from build123d import *

# Parameters (mm, degrees)
BOSS_EXTRUDE1_DEPTH = 15
BOSS_EXTRUDE2_DEPTH = 15
CUT_EXTRUDE1_DEPTH  = 14
SKETCH8_W           = 6.699223296
SKETCH8_H           = 4.721357371
SKETCH8_W_2         = 8.228893272
CUT_EXTRUDE7_DEPTH  = 3
SKETCH10_R          = 1.1
CUT_EXTRUDE9_DEPTH  = 15


with BuildPart() as part:
    # Sketch3 → Boss-Extrude1 (new body)
    with BuildSketch(Plane.XY.offset(1303.472903018)):
        with BuildLine():
            Line((787.650097371, 1035.49652121), (787.650097371, 1120.589424436))
            ThreePointArc((787.650097371, 1120.589424436), (788.529097371, 1122.710424436), (790.650097371, 1123.589424436))
            Line((790.650097371, 1123.589424436), (812.066097371, 1123.589424436))
            ThreePointArc((812.066097371, 1123.589424436), (814.187097371, 1122.710424436), (815.066097371, 1120.589424436))
            Line((815.066097371, 1120.589424436), (815.066097371, 1103.589424436))
            ThreePointArc((815.066097371, 1103.589424436), (815.945097371, 1101.468424436), (818.066097371, 1100.589424436))
            Line((818.066097371, 1100.589424436), (834.650097371, 1100.589424436))
            Line((834.650097371, 1100.589424436), (834.650461973, 1102.58942437))
            Line((834.650461973, 1102.58942437), (818.066461973, 1102.58942437))
            ThreePointArc((818.066461973, 1102.58942437), (817.35931084, 1102.882637905), (817.066097305, 1103.589789038))
            Line((817.066097305, 1103.589789038), (817.066097305, 1120.589789038))
            ThreePointArc((817.066097305, 1120.589789038), (815.601310896, 1124.124637961), (812.066461973, 1125.58942437))
            Line((812.066461973, 1125.58942437), (790.64973277, 1125.58942437))
            ThreePointArc((790.64973277, 1125.58942437), (787.114883847, 1124.124637961), (785.650097438, 1120.589789038))
            Line((785.650097438, 1120.589789038), (785.650097371, 1033.49652121))
            Line((785.650097371, 1033.49652121), (834.649003168, 1033.49652121))
            Line((834.649003168, 1033.49652121), (834.649003168, 1035.49652121))
            Line((834.649003168, 1035.49652121), (787.650097371, 1035.49652121))
        make_face()
    extrude(amount=BOSS_EXTRUDE1_DEPTH)

    # Sketch6 → Boss-Extrude2 (add)
    with BuildSketch(Plane.XY.offset(1303.472903018)):
        with BuildLine():
            Line((787.650097371, 1035.49652121), (834.649003168, 1035.49652121))
            Line((834.649003168, 1035.49652121), (844.649003168, 1035.49652121))
            Line((844.649003168, 1035.49652121), (844.650097371, 1100.589424436))
            Line((844.650097371, 1100.589424436), (834.650097371, 1100.589424436))
            Line((834.650097371, 1100.589424436), (818.066097371, 1100.589424436))
            ThreePointArc((818.066097371, 1100.589424436), (815.945097371, 1101.468424436), (815.066097371, 1103.589424436))
            Line((815.066097371, 1103.589424436), (815.066097371, 1120.589424436))
            ThreePointArc((815.066097371, 1120.589424436), (814.187097371, 1122.710424436), (812.066097371, 1123.589424436))
            Line((812.066097371, 1123.589424436), (790.650097371, 1123.589424436))
            ThreePointArc((790.650097371, 1123.589424436), (788.529097371, 1122.710424436), (787.650097371, 1120.589424436))
            Line((787.650097371, 1120.589424436), (787.650097371, 1035.49652121))
        make_face()
    extrude(amount=BOSS_EXTRUDE2_DEPTH)

    # Sketch6<2> → Cut-Extrude1 (cut)
    with BuildSketch(Plane.XY.offset(1303.472903018)):
        with BuildLine():
            Line((787.650097371, 1035.49652121), (834.649003168, 1035.49652121))
            Line((834.649003168, 1035.49652121), (844.649003168, 1035.49652121))
            Line((844.649003168, 1035.49652121), (844.650097371, 1100.589424436))
            Line((844.650097371, 1100.589424436), (834.650097371, 1100.589424436))
            Line((834.650097371, 1100.589424436), (818.066097371, 1100.589424436))
            ThreePointArc((818.066097371, 1100.589424436), (815.945097371, 1101.468424436), (815.066097371, 1103.589424436))
            Line((815.066097371, 1103.589424436), (815.066097371, 1120.589424436))
            ThreePointArc((815.066097371, 1120.589424436), (814.187097371, 1122.710424436), (812.066097371, 1123.589424436))
            Line((812.066097371, 1123.589424436), (790.650097371, 1123.589424436))
            ThreePointArc((790.650097371, 1123.589424436), (788.529097371, 1122.710424436), (787.650097371, 1120.589424436))
            Line((787.650097371, 1120.589424436), (787.650097371, 1035.49652121))
        make_face()
    extrude(amount=CUT_EXTRUDE1_DEPTH, mode=Mode.SUBTRACT)

    # Sketch8 → Cut-Extrude7 (cut)
    with BuildSketch(Plane.XY.offset(1303.472903018)):
        with Locations((788.177093813, 1120.255926572)):
            Rectangle(SKETCH8_W, SKETCH8_H)
        with Locations((813.958809837, 1120.255926572)):
            Rectangle(SKETCH8_W_2, SKETCH8_H)
    extrude(amount=CUT_EXTRUDE7_DEPTH, mode=Mode.SUBTRACT)

    # Sketch10 → Cut-Extrude9 (cut)
    with BuildSketch(Plane.XY.offset(1303.472903018)):
        with Locations((832.650097371, 1039.589424436)):
            Circle(SKETCH10_R)
        with Locations((792.650097371, 1039.589424436)):
            Circle(SKETCH10_R)
        with Locations((792.650097371, 1097.589424436)):
            Circle(SKETCH10_R)
        with Locations((812.650097371, 1097.589424436)):
            Circle(SKETCH10_R)
    extrude(amount=CUT_EXTRUDE9_DEPTH, mode=Mode.SUBTRACT)


solid = part.part
Could you check a few things on this model? Use its own coordinates, in mm. A direction names the side the tool comes from. Give positions to 0.01 mm unless a question says otherwise; leave off trailing zeros. Order: outer loops, then holes, each group sorted by start corner. A loop starts at its lowest first (then second) coordinate and runs counter-clockwise, first axis right, second up. Notation, with made-up numbers: (82, -16.75) - (100, -16.75) arc R24 cw to (100, 3.25) - close; hole circle Ø11 at (25, 9). An arc over 180 degrees is marked (long way). Return JSON: item names as keys, results as strings. Group by question number.
Q1. Will these pins go through, and if not, where does the flat tip stop? pin 1 Ø0.6 at (x, z) = (816, 1305.5) entering from +Y; pin 2 Ø0.8 at (x, y) = (787, 1119.5) entering from -Z; pin 3 Ø0.6 at (x, z) = (786.5, 1305) entering from +Y.
Q2. Suppose I cut it at B-B, the plane y = 1107.5. Please give me the cut outline in (x, z).
Q3. Thinking about a two-plate mould opening in Y: for faces 1 (the face through (826, 1102.589, 1311)), 2 (the face through (815, 1080, 1318.473)), 3 (the face through (816, 1120, 1306.473)), which applies, pulls with the +Y half, pulls with the -Y half, needs draft (parallel to the pull), parting line crosses it, or undercut?
Q4. Suppose I cut it at C-C, the plane z = 1311.75. Please give me the cut outline in (x, y) (3 decimals).
Q5. Suppose I cut it at A-A, the plane x = 808. Please give me the cut outline in (y, z).
Q6. Suppose I cut it at D-D, the plane y = 1073. Please give me the cut outline in (x, z).
Q7. Which directions (+Z, -Z, +X, -X, +Y, -Y) give clear straight access to the entire face, cutting with the end or side of a thin tool? Please do faces 4 (the face through (816, 1117.895, 1305)), 5 (the face through (826, 1100.589, 1310)), 6 (the face through (815.969, 1101.445, 1310.375)).
Q8. Please list where these lines run through material, in increasing order: line 1 along X through (y, z) = (1109, 1305); line 2 along Y through (x, z) = (811.5, 1313); line 3 along Z through (x, y) = (809.5, 1051.5). Write a range as [from, to].
Resolved:
{
 "1": {"pin 1": "stops at y = 1124.02", "pin 2": "stops at z = 1306.47", "pin 3": "stops at y = 1123.78"},
 "2": {"outline": "(785.65, 1303.47) - (787.65, 1303.47) - (787.65, 1317.47) - (815.07, 1317.47) - (815.07, 1303.47) - (817.07, 1303.47) - (817.07, 1318.47) - (785.65, 1318.47) - close"},
 "3": {"face 1": "pulls with the +Y half", "face 2": "needs draft", "face 3": "undercut"},
 "4": {"outline": "(785.65, 1033.497) - (834.649, 1033.497) - (834.649, 1035.497) - (787.65, 1035.497) - (787.65, 1120.589) arc R3.001 cw to (790.65, 1123.589) - (812.066, 1123.589) arc R3.001 cw to (815.066, 1120.589) - (815.066, 1103.589) arc R3.001 ccw to (818.066, 1100.589) - (834.65, 1100.589) - (834.65, 1102.589) - (818.066, 1102.589) arc R1.001 cw to (817.066, 1103.59) - (817.066, 1120.59) arc R5.001 ccw to (812.066, 1125.589) - (790.65, 1125.589) arc R5.001 ccw to (785.65, 1120.59) - close"},
 "5": {"outline": "(1033.5, 1303.47) - (1035.5, 1303.47) - (1035.5, 1317.47) - (1123.59, 1317.47) - (1123.59, 1303.47) - (1125.59, 1303.47) - (1125.59, 1318.47) - (1033.5, 1318.47) - close"},
 "6": {"outline": "(785.65, 1303.47) - (787.65, 1303.47) - (787.65, 1317.47) - (844.65, 1317.47) - (844.65, 1318.47) - (785.65, 1318.47) - close"},
 "7": {"face 4": "-Z, +X, -X", "face 5": "-Z, +X", "face 6": "-Z"},
 "8": {"line 1": "x = [785.65, 787.65], [815.07, 817.07]", "line 2": "y = [1033.5, 1035.5], [1123.59, 1125.59]", "line 3": "z = [1317.47, 1318.47]"}
}
